The model under review builds one solid part; all positions refer to its coordinate system, in mm. Give positions to 0.01 mm unless a question says otherwise; leave off trailing zeros. Loops run counter-clockwise (first coordinate to the right, second up) from the corner with the lowest first, then second, coordinate; pieces in that order, holes last. Notation, with made-up numbers: (62.25, 76.5) - (104.25, 76.5) arc R10 cw to (104.25, 91.5) - close; hole circle Ø6 at (-40, 83.5). An arc over 180 degrees is marked (long way). Answer as a JSON object with one key per item and string values.
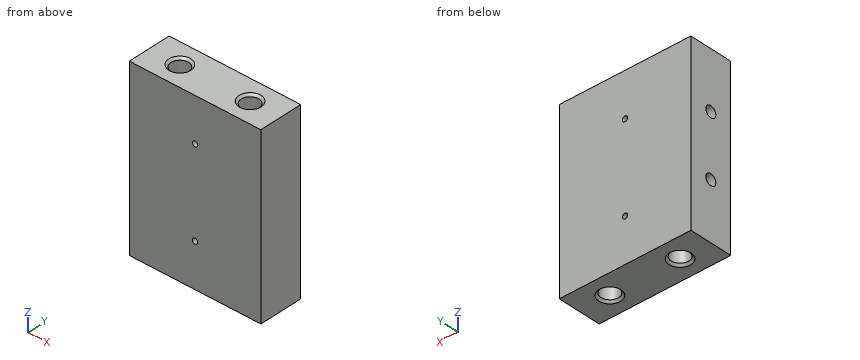
from build123d import *

# Parameters (mm, degrees)
SKETCH1_W                        = 38.1
SKETCH1_H                        = 12.7
BOSS_EXTRUDE1_DEPTH              = 50.8
F_1_4_20_TAPPED_HOLE1_AT_2_COUNT = 2
F_1_4_20_TAPPED_HOLE1_AT_2_PITCH = 20.32
F_1_64_TAPPED_HOLE1_D            = 1.5113
F_1_8_0_125_DIAMETER_HOLE1_D     = 3.175
F_1_8_0_125_DIAMETER_HOLE1_DEPTH = 5.08
F_1_8_0_125_DIAMETER_HOLE1_TIP   = 0.953866233


with BuildPart() as part:
    # Sketch1 → Boss-Extrude1 (new body)
    with BuildSketch(Plane.XY):
        Rectangle(SKETCH1_W, SKETCH1_H)
    extrude(amount=-BOSS_EXTRUDE1_DEPTH)

    # Sketch4 → 1/4-20 Tapped Hole1 (revolve, cut)
    with BuildSketch(Plane(origin=(-10.16, 0, 0), x_dir=(0, -1, 0), z_dir=(1, 0, 0))):
        Polygon((0, 0), (0, 14.233816902), (2.5527, 12.7), (2.5527, 0.635), (3.1877, 0), align=None)
    f_1_4_20_tapped_hole1 = revolve(axis=Axis((-10.16, 0, 6.35), (0, 0, -1)), mode=Mode.SUBTRACT)

    # 1/4-20 Tapped Hole1 at 2: 1/4-20 Tapped Hole1 ×2
    with Locations(*[(i * F_1_4_20_TAPPED_HOLE1_AT_2_PITCH, 0, 0) for i in range(1, F_1_4_20_TAPPED_HOLE1_AT_2_COUNT)]):
        add(f_1_4_20_tapped_hole1, mode=Mode.SUBTRACT)

    # Mirror1: 1/4-20 Tapped Hole1 across plane
    add(f_1_4_20_tapped_hole1.mirror(Plane.XY.offset(-25.4)), mode=Mode.SUBTRACT)

    # Mirror1 copy 1 sketch → Mirror1 copy 1 (revolve, cut)
    with BuildSketch(Plane(origin=(10.16, 0, -50.8), x_dir=(0, -1, 0), z_dir=(1, 0, 0))):
        Polygon((0, 0), (0, -14.233816902), (2.5527, -12.7), (2.5527, -0.635), (3.1877, 0), align=None)
    revolve(axis=Axis((10.16, 0, -57.15), (0, 0, -1)), mode=Mode.SUBTRACT)

    # #1-64 Tapped Hole1 (through all)
    with Locations(Plane(origin=(0, 6.35, -38.1), x_dir=(0, 0, 1), z_dir=(0, 1, 0))):
        with Locations((0, 0), (25.4, 0)):
            Hole(F_1_64_TAPPED_HOLE1_D / 2)

    # 1/8 (0.125) Diameter Hole1
    with Locations(Plane.ZY.offset(19.05)):
        with Locations((-34.29, 0), (-16.51, 0)):
            Hole(F_1_8_0_125_DIAMETER_HOLE1_D / 2, depth=F_1_8_0_125_DIAMETER_HOLE1_DEPTH)
            with Locations((0, 0, -(F_1_8_0_125_DIAMETER_HOLE1_DEPTH + F_1_8_0_125_DIAMETER_HOLE1_TIP / 2))):  # 118° drill point
                Cone(0, F_1_8_0_125_DIAMETER_HOLE1_D / 2, F_1_8_0_125_DIAMETER_HOLE1_TIP, mode=Mode.SUBTRACT)


solid = part.part
Q1. Consider section A-A, the plane x = 0. State the section outline as (y, z) points.
Results:
{"outline": "(-6.35, -50.8) - (6.35, -50.8) - (6.35, -38.86) - (-6.35, -38.86) - close; (-6.35, -37.34) - (6.35, -37.34) - (6.35, -13.46) - (-6.35, -13.46) - close; (-6.35, -11.94) - (6.35, -11.94) - (6.35, 0) - (-6.35, 0) - close"}
Q2. Clearance check with flat-ended pins moving along their axes: pin 1 Ø3 at (x, y) = (10.16, 0) entering from -Z; pin 2 Ø6 at (x, y) = (-10.16, 0) entering from +Z; pin 3 Ø3 at (x, y) = (-10.5, -0.5) entering from -Z. State where each tip first meets the part, or that it passes through.
Results:
{"pin 1": "stops at z = -37.47", "pin 2": "stops at z = -0.19", "pin 3": "stops at z = -37.83"}
Q3. To check wall thickness, follow probe 1 along Z at (x, y) = (-17.2, 0); probe 2 along X at (y, z) = (0, -8.25); probe 3 along Y at (x, z) = (-16.8, -16.51). State the ranges of each line that lie inside material, in increasing order. Write a range as [from, to].
Results:
{"probe 1": "z = [-50.8, -35.88], [-32.7, -18.1], [-14.92, 0]", "probe 2": "x = [-19.05, -12.71], [-7.61, 7.61], [12.71, 19.05]", "probe 3": "y = [-6.35, -1.59], [1.59, 6.35]"}
Q4. Consider section B-B, the plane z = -43. State the section outline as (x, y) points.
Results:
{"outline": "(-19.05, -6.35) - (19.05, -6.35) - (19.05, 6.35) - (-19.05, 6.35) - close; hole circle Ø5.11 at (-10.16, 0); hole circle Ø5.11 at (10.16, 0)"}
